Design review of the part shown in the three views and the two pictorial views. Dimensions are in mm from the part's minimum x, y and z. A direction names the side the tool comes from. Round coordinates to 2 decimals unless told otherwise and drop trailing zeros. Loops run counter-clockwise (first coordinate to the right, second up) from the corner with the lowest first, then second, coordinate; pieces in that order, holes last. Notation, with made-up numbers: M -23,-22 L -1,-22 A30 cw -1,10 Z; hole C 61.25,43 d9. An arc over 180 degrees is marked long. Return JSON: item names as keys, results as strings. Group by question number.
Q1. Consider section C-C (y = 19.25). State the section outline as (x, z) points, and give its area (3 significant figures).
Q2. Draft analysis for pull direction Z (two halves, no side actions). For the marked faces 4, 5 and 6, state which applies: pulls with the +Z half, pulls with the -Z half, needs draft (parallel to the pull), parting line crosses it, or undercut.
Q3. Consider section B-B (z = 25.5). State the section outline as (x, y) points.
Q4. Consider section D-D (z = 36). State the section outline as (x, y) points.
Q5. For the marked faces 1, 2 and 3, list the 3-axis set-ups (+Z, -Z, +X, -X, +Y, -Y) from which the entire face can be reached by the end or side of a thin tool; tool diameter is ignored.
Q6. To check wall thickness, follow line 1 along Z through (x, y) = (25.5, 19.75); line 2 along Z through (x, y) = (25.5, 7.75); line 3 along Y through (x, z) = (6.5, 40.5). State the ranges of each line that lie inside material, in increasing order.
Q7. Clearance check with flat-ended pins moving along their axes: pin 1 Ø4 at (x, z) = (6, 16) entering from -Y; pin 2 Ø10 at (x, z) = (32.5, 37) entering from -Y; pin 3 Ø12 at (y, z) = (3, 44) entering from -X. State where each tip first meets the part, or that it passes through.
Q8. Consider section A-A (x = 25.5). State the section outline as (y, z) points.
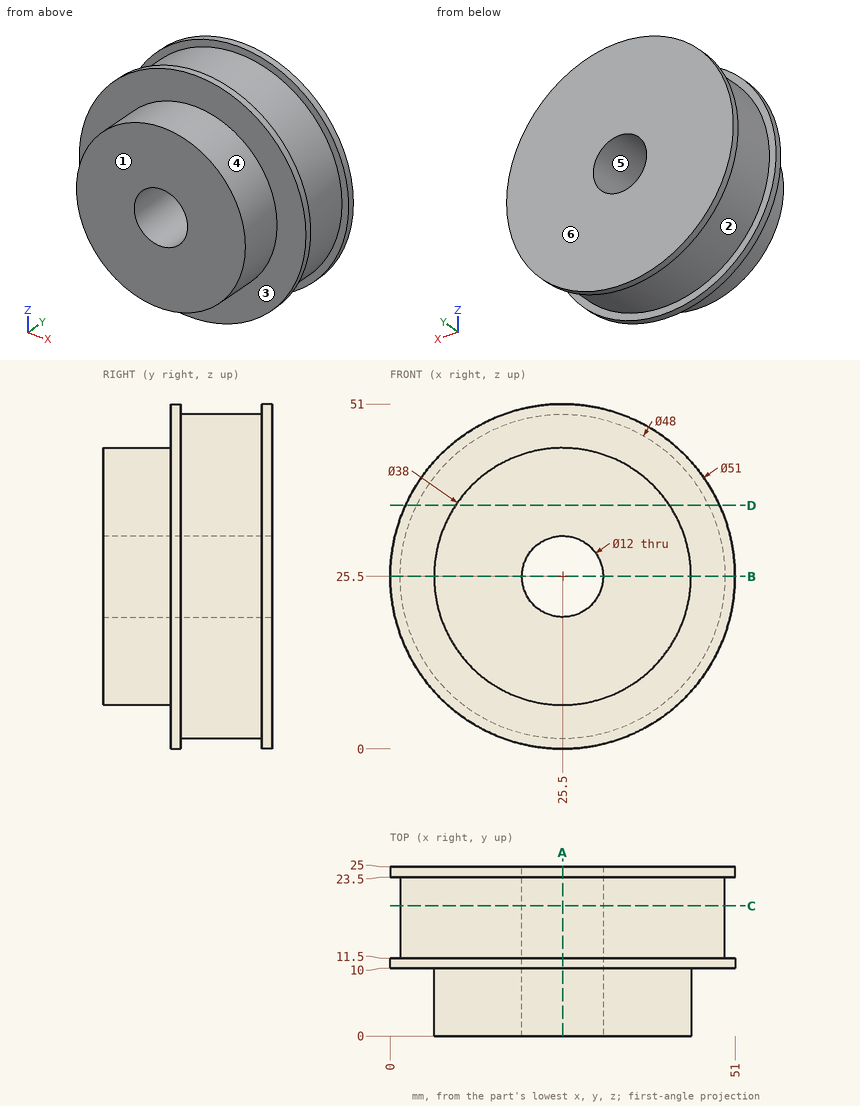
Values:
{
 "1": {"outline": "C 25.5,25.5 d48; hole C 25.5,25.5 d12", "area": "1,700 mm2"},
 "2": {"face 4": "parting line crosses it", "face 5": "undercut", "face 6": "needs draft"},
 "3": {"outline": "M 0,10 L 6.5,10 L 6.5,0 L 19.5,0 L 19.5,25 L 0,25 L 0,23.5 L 1.5,23.5 L 1.5,11.5 L 0,11.5 Z; M 31.5,0 L 44.5,0 L 44.5,10 L 51,10 L 51,11.5 L 49.5,11.5 L 49.5,23.5 L 51,23.5 L 51,25 L 31.5,25 Z"},
 "4": {"outline": "M 2.26,10 L 9.66,10 L 9.66,0 L 41.34,0 L 41.34,10 L 48.74,10 L 48.74,11.5 L 47.08,11.5 L 47.08,23.5 L 48.74,23.5 L 48.74,25 L 2.26,25 L 2.26,23.5 L 3.92,23.5 L 3.92,11.5 L 2.26,11.5 Z"},
 "5": {"face 1": "+Z, -Z, +X, -X, -Y", "face 2": "none", "face 3": "-Y"},
 "6": {"line 1": "z = 1.5 to 19.5, 31.5 to 49.5", "line 2": "z = 6.5 to 19.5, 31.5 to 44.5", "line 3": "y = 10 to 11.5, 23.5 to 25"},
 "7": {"pin 1": "stops at y = 10", "pin 2": "stops at y = 0", "pin 3": "stops at x = 11.19"},
 "8": {"outline": "M 0,6.5 L 10,6.5 L 10,0 L 11.5,0 L 11.5,1.5 L 23.5,1.5 L 23.5,0 L 25,0 L 25,19.5 L 0,19.5 Z; M 0,31.5 L 25,31.5 L 25,51 L 23.5,51 L 23.5,49.5 L 11.5,49.5 L 11.5,51 L 10,51 L 10,44.5 L 0,44.5 Z"}
}
